Geometry check sheet. Reference: the model listing, model coordinates, mm. Face numbers are marked on the shaded views. A direction names the side the tool comes from. Give positions to 0.01 mm unless a question says otherwise; leave off trailing zeros. Write each loop counter-clockwise with the first axis right and the second up, starting at its lowest first coordinate (ties: lowest second). Pieces come first, ordered by that corner, then holes.
(1) Tool access check on the marked faces 5 and 6. Record the directions out of +Z, -Z, +X, -X, +Y, -Y that give a thin tool (end or side, any length) a straight path to the whole face; none if there is none.
(2) Cross-section at B-B (x = -33). Record the boundary of the cut face in (y, z).
(3) Mould release check, pull along Y, two halves, no side actions. Record for the marked faces 1, 2, 3 and 4: +Y half, -Y half, draft (parallel to the pull), parting line (faces both ways), or undercut.
(4) Depth check by flat-ended pin: P1, Ø8, axis at x = -39.5, z = 0, coming from the +Y side; P2, Ø1.5, axis at x = -44.5, z = 4.5, coming from the -Y side; P3, Ø4, axis at x = -47.5, z = 3, coming from the -Y side. Enter the tip coordinate at first touch or a pass-through.
(5) Cross-section at C-C (x = -60). Record the boundary of the cut face in (y, z), and give its area (3 significant figures).
(6) Thickness scan on line 1 along X through (y, z) = (6.5, 2); line 2 along Y through (x, z) = (-49, 0.25). Record the ranges inside material, lowest first.
(7) Cross-section at A-A (y = 0). Record the boundary of the cut face in (x, z), and give its area (3 significant figures).
Autodesk Inventor part; units mm, degrees
ref_plane "YZ Plane" through (0, 0, 0) normal (1, 0, 0) x (0, 1, 0)
ref_plane "XZ Plane" through (0, 0, 0) normal (0, 1, 0) x (-1, 0, 0)
ref_plane "XY Plane" through (0, 0, 0) normal (0, 0, 1) x (1, 0, 0)
sketch "Sketch1" plane through (0, 0, 0) normal (0, 0, 1) x (1, 0, 0)
  line L0 (0, 0) -> (-81, 0)
  line L1 (-81, 0) -> (-81, 5)
  line L2 (-81, 5) -> (-75, 5)
  line L3 (-75, 5) -> (-75, 7)
  line L4 (-75, 7) -> (-35, 7)
  line L5 (-35, 7) -> (-25, 10.5)
  line L6 (-25, 10.5) -> (0, 10.5)
  line L7 (0, 10.5) -> (0, 0)
  line L8 (-97.2, 0) -> (16.2, 0)
  dimension "d7" = 5
  dimension "d8" = 6
  dimension "d9" = 7
  dimension "d10" = 25
  dimension "d11" = 50
  dimension "d12" = 10
  dimension "d13" = 10.5
revolve "Revolution1" add sketch "Sketch1" angle 360 about axis through (-10, 0, 0) along (1, 0, 0)
thread "Thread1"
sketch "Sketch2" plane through (0, 0, 0) normal (1, 0, 0) x (0, 0, -1)
  circle A0 centre (0, 0) radius 10.5
  line L0 (-7.4246, -7.4246) -> (7.4246, -7.4246)
  line L1 (7.4246, -7.4246) -> (7.4246, 7.4246)
  line L2 (7.4246, 7.4246) -> (-7.4246, 7.4246)
  line L3 (-7.4246, 7.4246) -> (-7.4246, -7.4246)
  line L4 (-7.4246, -7.4246) -> (7.4246, 7.4246) construction
  line L5 (7.4246, -7.4246) -> (-7.4246, 7.4246) construction
  circle A1 centre (0, 0) radius 20.6149
extrude "Extrusion1" cut sketch "Sketch2" against normal up to next contours A0 L1 | L2 A0 | A0 L0 | L3 A0 | A1
properties part number "tool clamping screw"
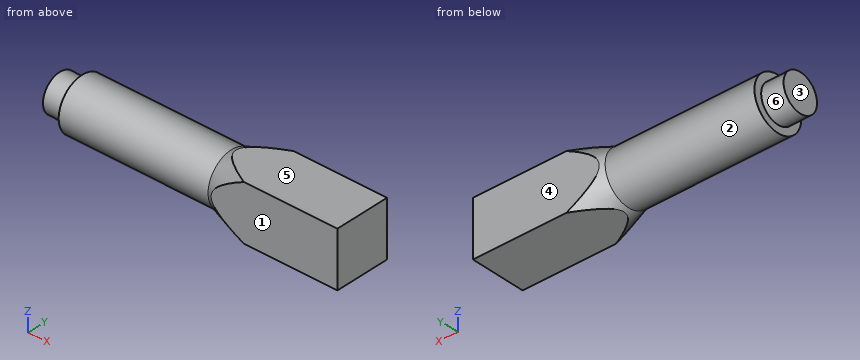
Reply:
1. face 5: +Z, +X, -X, +Y, -Y
1. face 6: -X
2. outline: (-7.42, -2.04) arc R7.7 ccw to (-2.04, -7.42) - (2.04, -7.42) arc R7.7 ccw to (7.42, -2.04) - (7.42, 2.04) arc R7.7 ccw to (2.04, 7.42) - (-2.04, 7.42) arc R7.7 ccw to (-7.42, 2.04) - close
3. face 1: -Y half
3. face 2: parting line
3. face 3: draft
3. face 4: +Y half
4. P1: stops at y = 7
4. P2: stops at y = -5.91
4. P3: stops at y = -6.93
5. outline: circle Ø14 at (0, 0)
5. area: 154 mm2
6. line 1: x = -75 to 0
6. line 2: y = -7 to 7
7. outline: (-81, -5) - (-75, -5) - (-75, -7) - (-35, -7) - (-33.79, -7.42) - (0, -7.42) - (0, 7.42) - (-33.79, 7.42) - (-35, 7) - (-75, 7) - (-75, 5) - (-81, 5) - close
7. area: 1,140 mm2
